CAD build for the part. Positions are in the model's coordinates, mm. A direction names the side the tool comes from. Coordinates: 2 decimals unless noted, no trailing zeros. Loops run counter-clockwise (first coordinate to the right, second up) from the corner with the lowest first, then second, coordinate; pieces in that order, holes last.
1) Saw through at B-B, the plane x = 26. Write the cut outline in (y, z).
2) Saw through at A-A, the plane x = 12. Write the cut outline in (y, z).
3) Pin check, flat tips, straight feed: pin 1 Ø0.8 at (y, z) = (0.5, 1) entering from -X; pin 2 Ø2 at (x, y) = (22, 0) entering from -Z; pin 3 Ø0.5 at (x, y) = (0.5, 0.5) entering from +Z. Stop position of each tip, or through.
4) Wall check: line 1 along X through (y, z) = (-2.5, -1.5); line 2 along X through (y, z) = (-4.5, -1.5); line 3 along X through (y, z) = (0.5, 2). Give the ranges that are in metal, low to high.
5) Two-plate mould, pull along Z, no slides. Class faces 1 (the flat face through (1, 0, 1.54)), 2 (the flat face through (4.5, 3.3, -1)), 3 (the cylindrical face through (5.72, -2.35, -1.8)), 4 (the flat face through (1.18, -1.33, 0.78)): +Z half, -Z half, draft (parallel to the pull), parting line (faces both ways), or undercut.
6) Which spindle directions (+Z, -Z, +X, -X, +Y, -Y) get a long thin tool onto all of the face, cutting with end or side? Do faces 5 (the flat face through (30.25, 0, 0)), 6 (the cylindrical face through (22.042, -0.24, 1.824)), 7 (the cylindrical face through (13.844, -0.703, -3.166)), 8 (the flat face through (1, 0, -1.54)), 9 (the flat face through (0, 0, -2)). Say none if no direction does.
```python
from build123d import *

# Parameters (mm, degrees)
CHAMFER1_SIZE = 0.2
HEX_2_DEPTH   = 2.4


# Read off the part's stored shape, not the designer's step: ThreadSchematic
with BuildPart() as part:
    # ThreadSchematic outline → ThreadSchematic (revolve)
    with BuildSketch(Plane.YX):
        with BuildLine():
            Line((0, 30.25), (0, 0))
            Line((0, 0), (5, 0))
            Line((5, 0), (5, 4.5))
            Line((5, 4.5), (3.16, 4.5))
            ThreePointArc((3.16, 4.5), (3.018578644, 4.558578644), (2.96, 4.7))
            Line((2.96, 4.7), (2.96, 6.7165))
            Line((2.96, 6.7165), (3.2435, 7))
            Line((3.2435, 7), (3.2435, 20.5))
            Line((3.2435, 20.5), (2.5, 20.5))
            ThreePointArc((2.5, 20.5), (2.033309524, 20.693309524), (1.84, 21.16))
            Line((1.84, 21.16), (1.84, 22.9))
            Line((1.84, 22.9), (2.5, 23.56))
            Line((2.5, 23.56), (2.5, 29.805))
            Line((2.5, 29.805), (2.055, 30.25))
            Line((2.055, 30.25), (0, 30.25))
        make_face()
    revolve(axis=Axis((0, 0, 0), (1, 0, 0)))

    # Chamfer1
    chamfer1_edges = [part.edges().sort_by_distance(p)[0] for p in [
        (0, -5, 0),
    ]]
    chamfer(chamfer1_edges, length=CHAMFER1_SIZE)

    # Sketch2 → PreBroach (revolve, cut)
    with BuildSketch(Plane.XY, mode=Mode.PRIVATE) as prebroach_sk:
        Polygon((0, 1.54), (2.4, 1.54), (3.289119415, 0), (0, 0), align=None)
    revolve(prebroach_sk.sketch.rotate(Axis((0, 0, 0), (1, 0, 0)), 90), axis=Axis((0, 0, 0), (1, 0, 0)), mode=Mode.SUBTRACT)

    # Sketch3 → Hex 2 (cut)
    with BuildSketch(Plane.ZY):
        Polygon((-1.54, -0.889119415), (-1.54, 0.889119415), (0, 1.778238829), (1.54, 0.889119415), (1.54, -0.889119415), (0, -1.778238829), align=None)
    extrude(amount=-HEX_2_DEPTH, mode=Mode.SUBTRACT)


solid = part.part
```
Data:
1. outline: circle Ø5 at (0, 0)
2. outline: circle Ø6.49 at (0, 0)
3. pin 1: stops at x = 2.41
3. pin 2: stops at z = -1.94
3. pin 3: stops at z = 4.99
4. line 1: x = 0 to 20.5
4. line 2: x = 0 to 4.5
4. line 3: x = 0 to 20.67, 23.12 to 30.24
5. face 1: undercut
5. face 2: draft
5. face 3: parting line
5. face 4: undercut
6. face 5: +Z, -Z, +X, +Y, -Y
6. face 6: none
6. face 7: +X
6. face 8: -X
6. face 9: +Z, -Z, -X, +Y, -Y
